Input: part model. Units: mm. Frame: model coordinates. A direction names the side the tool comes from. Give positions to 0.01 mm unless a question says otherwise; leave off trailing zeros. Order: outer loops, then holes, each group sorted by start corner. A loop starts at its lowest first (then second) coordinate and runs counter-clockwise, first axis right, second up. Notation, with made-up numbers: M 32,-27.75 L 76,-27.75 A9 cw 76,-19.75 Z; hole C -35,84 d2. An arc over 180 degrees is marked long. Use a Markdown table: item, result.
from build123d import *

# Parameters (mm, degrees)
SKETCH_W        = 12
SKETCH_H        = 91.6
PAD_DEPTH       = 10
SKETCH001_R     = 2.65
POCKET_DEPTH    = 195.845666
POCKET001_DEPTH = 4.5
SKETCH003_R     = 5
POCKET002_DEPTH = 4.5
SKETCH004_R     = 2.6
POCKET003_DEPTH = 10.001
FILLET_R        = 2
CHAMFER_SIZE    = 1


with BuildPart() as part:
    # Sketch → Pad (new body)
    with BuildSketch(Plane.XY):
        Rectangle(SKETCH_W, SKETCH_H)
    extrude(amount=PAD_DEPTH)

    # Sketch001 (on Face6 of Pad) → Pocket (cut, through all)
    with BuildSketch(Plane.XY.offset(10)):
        with Locations((0, 27)):
            Circle(SKETCH001_R)
    pocket = extrude(amount=-POCKET_DEPTH, mode=Mode.SUBTRACT)

    # Sketch002 (on Face4 of Pocket) → Pocket001 (cut)
    with BuildSketch(Plane(origin=(0, 0, 0), x_dir=(1, 0, 0), z_dir=(0, 0, -1))):
        Polygon((0, -22.323463), (-4.05, -24.661731), (-4.05, -29.338269), (0, -31.676537), (4.05, -29.338269), (4.05, -24.661731), align=None)
    pocket001 = extrude(amount=-POCKET001_DEPTH, mode=Mode.SUBTRACT)

    # Mirrored: Pocket001, Pocket across XZ
    add(pocket001.mirror(Plane.XZ), mode=Mode.SUBTRACT)
    add(pocket.mirror(Plane.XZ), mode=Mode.SUBTRACT)

    # Sketch003 (on Face5 of Mirrored) → Pocket002 (cut)
    with BuildSketch(Plane.XY.offset(10)):
        with Locations((0, 17)):
            Circle(SKETCH003_R)
        with Locations((0, -37)):
            Circle(SKETCH003_R)
    extrude(amount=-POCKET002_DEPTH, mode=Mode.SUBTRACT)

    # Sketch004 (on Face5 of Pocket002) → Pocket003 (cut, through all)
    with BuildSketch(Plane.XY.offset(10)):
        with Locations((0, 17)):
            Circle(SKETCH004_R)
        with Locations((0, -37)):
            Circle(SKETCH004_R)
    extrude(amount=-POCKET003_DEPTH, mode=Mode.SUBTRACT)

    # Fillet
    fillet_edges = [part.edges().sort_by_distance(p)[0] for p in [
        (-6, 45.8, 5),
        (-6, -45.8, 5),
        (6, -45.8, 5),
        (6, 45.8, 5),
    ]]
    fillet(fillet_edges, radius=FILLET_R)

    # Chamfer
    chamfer_edges = [part.edges().sort_by_distance(p)[0] for p in [
        (-2.65, 27, 4.5),
        (-2.65, -27, 4.5),
    ]]
    chamfer(chamfer_edges, length=CHAMFER_SIZE)


solid = part.part
1) Material intervals for line 1 (Y direction, x = 3.5, z = 3); line 2 (Y direction, x = 0, z = 1.8); line 3 (Y direction, x = 0, z = 8.3), sorted ascending. Write a range as from..to.
Response values:
| item | result |
|---|---|
| line 1 | y = -45.8..-29.66, -24.34..24.34, 29.66..45.8 |
| line 2 | y = -45.8..-39.6, -34.4..-31.68, -22.32..14.4, 19.6..22.32, 31.68..45.8 |
| line 3 | y = -45.8..-42, -32..-29.65, -24.35..12, 22..24.35, 29.65..45.8 |
2) Mould query, pull axis X, two halves, no side actions, for faces 4 (the face through (0, 1, 10)), 5 (the face through (2, -30.52, 2.22)), 6 (the face through (5.4, -45.23, 5.07)). Classes: released by +X, released by -X, zero draft, split by the parting line, or undercut.
Response values:
| item | result |
|---|---|
| face 4 | zero draft |
| face 5 | undercut |
| face 6 | released by +X |
3) Cut plane B-B on z = 3.5. Return loops of the section in (x, y).
Response values:
| item | result |
|---|---|
| outline | M -6,-43.8 A2 ccw -4,-45.8 L 4,-45.8 A2 ccw 6,-43.8 L 6,43.8 A2 ccw 4,45.8 L -4,45.8 A2 ccw -6,43.8 Z; hole M -4.05,-29.34 L 0,-31.68 L 4.05,-29.34 L 4.05,-24.66 L 0,-22.32 L -4.05,-24.66 Z; hole M -4.05,24.66 L 0,22.32 L 4.05,24.66 L 4.05,29.34 L 0,31.68 L -4.05,29.34 Z; hole C 0,-37 d5.2; hole C 0,17 d5.2 |
4) Reachability of faces 1 (the face through (-2.053, 30.491, 2.218)), 2 (the face through (5.4, 45.23, 5.07)), 3 (the face through (2, -39, 5.5)) from +Z, -Z, +X, -X, +Y, -Y: full face, straight path, thin tool, end or side. Return the list, or none.
Response values:
| item | result |
|---|---|
| face 1 | -Z |
| face 2 | +Z, -Z, +X, +Y |
| face 3 | +Z |
5) Cut plane C-C on z = 9.25. Return loops of the section in (x, y), and give its area (3 significant figures).
Response values:
| item | result |
|---|---|
| outline | M -6,-43.8 A2 ccw -4,-45.8 L 4,-45.8 A2 ccw 6,-43.8 L 6,43.8 A2 ccw 4,45.8 L -4,45.8 A2 ccw -6,43.8 Z; hole C 0,-37 d10; hole C 0,17 d10; hole C 0,-27 d5.3; hole C 0,27 d5.3 |
| area | 895 mm² |
6) Cut plane D-D on x = 1. State how many separate pieces and enclosed holes the cut face has, and give its area (3 significant figures).
Response values:
| item | result |
|---|---|
| separate pieces | 5 |
| enclosed holes | 0 |
| area | 645 mm² |
7) Cut plane A-A on y = -27. Return loops of the section in (x, z), and give its area (3 significant figures).
Response values:
| item | result |
|---|---|
| outline | M -6,0 L -4.05,0 L -4.05,4.5 L -3.65,4.5 L -2.65,5.5 L -2.65,10 L -6,10 Z; M 2.65,5.5 L 3.65,4.5 L 4.05,4.5 L 4.05,0 L 6,0 L 6,10 L 2.65,10 Z |
| area | 53.4 mm² |
8) First-contact query: pin 1 Ø4.5 at (x, y) = (0, 17) entering from +Z; pin 2 Ø6 at (x, y) = (0, -27) entering from -Z. Flat tips, straight axial feed; report the tip coordinate or a pass-through.
Response values:
| item | result |
|---|---|
| pin 1 | passes through |
| pin 2 | stops at z = 5.15 |
